Geometry check sheet. Reference: the model listing, model coordinates, mm. Give positions to 0.01 mm unless a question says otherwise; leave off trailing zeros. Write each loop counter-clockwise with the first axis right and the second up, starting at its lowest first coordinate (ties: lowest second). Pieces come first, ordered by that corner, then holes. Notation, with made-up numbers: M -19,47.5 L 1,47.5 A32 cw 1,83.5 Z; hole C 30.25,-35.75 d2. An arc over 180 degrees is marked long. One line per item, written item: value. Start each with the question number.
1. Gauge pin test, flat end, axial feed: pin 1 (3 mm diameter, centred on x = -96, y = 83, fed in from +Z). Record the tip position at first contact, or that the pin passes through.
2. Scan lines: line 1 (X direction, y = 4, z = 1.15); line 2 (Y direction, x = -137.5, z = 1.9); line 3 (Y direction, x = -92, z = 0.45). Record each from-to range of solid material in increasing order.
3. Cross-section at A-A on y = 4. Record the cut outline in (x, z), then the cut area to 3 significant figures.
4. Cross-section at B-B on x = -96. Record the cut outline in (y, z), then the cut area to 3 significant figures.
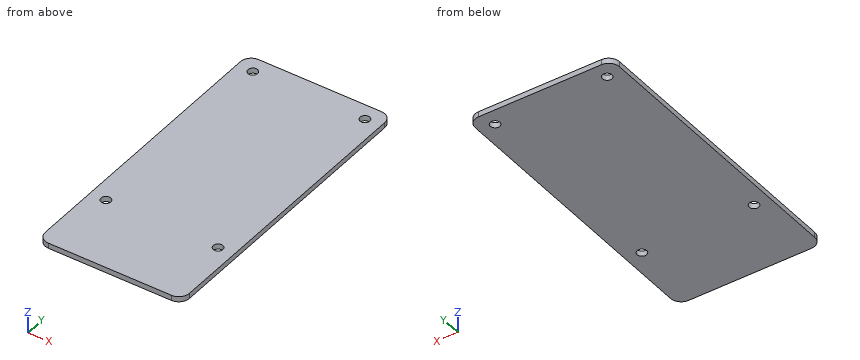
from build123d import *

# Parameters (mm, degrees)
BOSS_EXTRUDE1_DEPTH     = 2
SKETCH2_R               = 1.8
CUT_EXTRUDE1_DEPTH      = 1
CUT_EXTRUDE1_DEPTH_BACK = 15.56824426


with BuildPart() as part:
    # Sketch1 → Boss-Extrude1 (new body)
    with BuildSketch(Plane.XY):
        with BuildLine():
            Line((-140.00000048, 89.00000126), (-93.99999888, 89.00000126))
            ThreePointArc((-93.99999888, 89.00000126), (-91.171571755, 87.828428385), (-89.99999888, 85.00000126))
            Line((-89.99999888, 85.00000126), (-89.99999888, -19.99999918))
            ThreePointArc((-89.99999888, -19.99999918), (-91.171571755, -22.828426305), (-93.99999888, -23.99999918))
            Line((-93.99999888, -23.99999918), (-140.00000048, -23.99999918))
            ThreePointArc((-140.00000048, -23.99999918), (-142.828427605, -22.828426305), (-144.00000048, -19.99999918))
            Line((-144.00000048, -19.99999918), (-144.00000048, 85.00000126))
            ThreePointArc((-144.00000048, 85.00000126), (-142.828427605, 87.828428385), (-140.00000048, 89.00000126))
        make_face()
    extrude(amount=BOSS_EXTRUDE1_DEPTH)

    # Sketch2 → Cut-Extrude1 (cut, two sides)
    with BuildSketch(Plane(origin=(0, 0, -12.56824426), x_dir=(-1, 0, 0), z_dir=(0, 0, -1))) as cut_extrude1_sk:
        with Locations((95.9999985, 82.99999962)):
            Circle(SKETCH2_R)
        with Locations((137.9999985, 82.99999962)):
            Circle(SKETCH2_R)
        with Locations((137.9999985, 3.99999962)):
            Circle(SKETCH2_R)
        with Locations((95.9999985, 3.99999962)):
            Circle(SKETCH2_R)
    extrude(amount=CUT_EXTRUDE1_DEPTH, mode=Mode.SUBTRACT)
    extrude(cut_extrude1_sk.sketch, amount=-CUT_EXTRUDE1_DEPTH_BACK, mode=Mode.SUBTRACT)


solid = part.part
Report:
1. pin 1: passes through
2. line 1: x = -144 to -139.8, -136.2 to -97.8, -94.2 to -90
2. line 2: y = -24 to 2.27, 5.73 to 81.27, 84.73 to 89
2. line 3: y = -23.46 to 88.46
3. outline: M -144,0 L -139.8,0 L -139.8,2 L -144,2 Z; M -136.2,0 L -97.8,0 L -97.8,2 L -136.2,2 Z; M -94.2,0 L -90,0 L -90,2 L -94.2,2 Z
3. area: 93.6 mm^2
4. outline: M -24,0 L 2.2,0 L 2.2,2 L -24,2 Z; M 5.8,0 L 81.2,0 L 81.2,2 L 5.8,2 Z; M 84.8,0 L 89,0 L 89,2 L 84.8,2 Z
4. area: 212 mm^2
